For this review, take the finished solid that the model builds, in its own axes (mm). A direction names the side the tool comes from. Coordinates: 2 decimals unless noted, no trailing zeros. Loops run counter-clockwise (first coordinate to the right, second up) from the corner with the lowest first, then second, coordinate; pieces in that order, holes last. Notation, with made-up numbers: (87, -8) - (98, -8) arc R24 ccw to (98, 10) - close; hole circle Ø3 at (44.25, -9.75). An arc over 180 degrees is marked (long way). Answer as a JSON object with one key per item and string values. Group by question number.
Item 1: We need section A-A (x = 0). Give the boundary of the cut face in (y, z), then the cut area to 3 significant figures.
Item 2: We need section D-D (z = 4.5). Give the boundary of the cut face in (x, y), then the cut area to 3 significant figures.
Item 3: Mouldability with a two-part tool opening along Z and no side actions: class faces 1 (the cylindrical face through (-3.905, 9.126, -0.867)), 2 (the flat face through (2, 17, 6)), 3 (the cylindrical face through (2.703, 17.493, 8.584)) as released by +Z, released by -Z, zero draft, split by the parting line, or undercut.
Item 4: Clearance check with flat-ended pins moving along their axes: pin 1 (4 mm diameter, centred on y = 5.5, z = -2.5, fed in from -X); pin 2 (3 mm diameter, centred on y = 4.5, z = 3, fed in from +X); pin 3 (6 mm diameter, centred on y = 11.5, z = 5, fed in from -X). State where each tip first meets the part, or that it passes through.
Item 5: To check wall thickness, follow line 1 (X direction, y = 11.25, z = 0); line 2 (X direction, y = 8.25, z = 0); line 3 (Y direction, x = 4, z = -6.5). State the ranges of each line that lie inside material, in increasing order.
Item 6: We need section B-B (z = 0). Give the boundary of the cut face in (x, y), then the cut area to 3 significant figures.
Item 7: Tool access review of faces 4 (the flat face through (-2, 18, 4)), 5 (the flat face through (2, 10, 6)): name each direction out of +Z, -Z, +X, -X, +Y, -Y from which nothing blocks a thin tool from reaching the whole face with its end or side.
Item 8: We need section C-C (y = 7.75). Give the boundary of the cut face in (x, z), then the cut area to 3 significant figures.
from build123d import *

# Parameters (mm, degrees)
SKETCH1_R           = 9
BOSS_EXTRUDE1_DEPTH = 18
SKETCH2_R           = 4
CUT_EXTRUDE1_DEPTH  = 23.045407685
CUT_EXTRUDE2_START  = -1
SKETCH3_R           = 10
SKETCH3_R_2         = 6
CUT_EXTRUDE2_DEPTH  = 7


with BuildPart() as part:
    # Sketch1 → Boss-Extrude1 (new body)
    with BuildSketch(Plane(origin=(0, 0, 0), x_dir=(1, 0, 0), z_dir=(0, 1, 0))):
        with Locations(Location((0, 0, 0), (0, 0, 270))):
            Circle(SKETCH1_R)
    extrude(amount=BOSS_EXTRUDE1_DEPTH)

    # Sketch2 → Cut-Extrude1 (cut, through all)
    with BuildSketch(Plane(origin=(0, 18, 0), x_dir=(1, 0, 0), z_dir=(0, 1, 0))):
        with Locations(Location((0, 0, 0), (0, 0, 270))):
            Circle(SKETCH2_R)
    extrude(amount=-CUT_EXTRUDE1_DEPTH, mode=Mode.SUBTRACT)

    # Sketch3 → Cut-Extrude2 (cut)
    with BuildSketch(Plane(origin=(0, 18, 0), x_dir=(1, 0, 0), z_dir=(0, 1, 0)).offset(CUT_EXTRUDE2_START)):
        Circle(SKETCH3_R)
        with Locations(Location((0, 0, 0), (0, 0, 270))):
            Circle(SKETCH3_R_2, mode=Mode.SUBTRACT)
    extrude(amount=-CUT_EXTRUDE2_DEPTH, mode=Mode.SUBTRACT)


solid = part.part
Check sheet entries:
{
 "1": {"outline": "(0, -9) - (10, -9) - (10, -6) - (17, -6) - (17, -9) - (18, -9) - (18, -4) - (0, -4) - close; (0, 4) - (18, 4) - (18, 9) - (17, 9) - (17, 6) - (10, 6) - (10, 9) - (0, 9) - close", "area": "138 mm2"},
 "2": {"outline": "(-7.79, 0) - (7.79, 0) - (7.79, 10) - (3.97, 10) - (3.97, 17) - (7.79, 17) - (7.79, 18) - (-7.79, 18) - (-7.79, 17) - (-3.97, 17) - (-3.97, 10) - (-7.79, 10) - close", "area": "227 mm2"},
 "3": {"face 1": "undercut", "face 2": "zero draft", "face 3": "split by the parting line"},
 "4": {"pin 1": "stops at x = -8.99", "pin 2": "stops at x = 8.87", "pin 3": "stops at x = -8.67"},
 "5": {"line 1": "x = -6 to -4, 4 to 6", "line 2": "x = -9 to -4, 4 to 9", "line 3": "y = 0 to 10, 17 to 18"},
 "6": {"outline": "(-9, 0) - (-4, 0) - (-4, 18) - (-9, 18) - (-9, 17) - (-6, 17) - (-6, 10) - (-9, 10) - close; (4, 0) - (9, 0) - (9, 10) - (6, 10) - (6, 17) - (9, 17) - (9, 18) - (4, 18) - close", "area": "138 mm2"},
 "7": {"face 4": "+Z, -Z, +X, -X, +Y", "face 5": "none"},
 "8": {"outline": "circle Ø18 at (0, 0); hole circle Ø8 at (0, 0)", "area": "204 mm2"}
}
